Input: part model. Units: mm. Frame: model coordinates. A direction names the side the tool comes from. Round coordinates to 2 decimals unless told otherwise and drop trailing zeros. Loops run counter-clockwise (first coordinate to the right, second up) from the corner with the lowest first, then second, coordinate; pieces in that order, holes last. Notation, with made-up numbers: M 24,-25 L 73,-25 A27 cw 73,11 Z; hole C -37.5,82 d1. An arc over 180 degrees is marked long. Put each result on its own line as item: value. Start each with the question number.
1) Section C-C on x = 77.5. Output: boundary loops of the cut face in (y, z), plus the area to 3 significant figures.
2) Reachability of faces 1 (the face through (19, 30, 21.59)), 2 (the face through (0, 20, 0)), 3 (the face through (23, 32.283, -4)), 4 (the face through (95, 30, -21.59)) from +Z, -Z, +X, -X, +Y, -Y: full face, straight path, thin tool, end or side. Return the list, or none.
3) Draft query along Y for faces 5 (the face through (91.58, 34.45, 4.73)), 6 (the face through (57, -2.82, 8)), 7 (the face through (95, 27.914, 0)). Return one class per face: +Y half, -Y half, draft (parallel to the pull), parting line (faces both ways), or undercut.
4) Line query: probe 1 along Z at (x, y) = (25, 17); probe 2 along Z at (x, y) = (29, 28.5); probe 3 along Y at (x, z) = (96, -24). Output: solid intervals per line, ascending.
5) Section D-D on x = 39.5. Output: boundary loops of the cut face in (y, z).
6) Pin query (flat end, axial travel): pin 1 (19 mm diameter, centred on x = 88.9, z = 0, fed in from -Y); pin 2 (6.5 mm diameter, centred on x = 88.9, z = 0, fed in from +Y) (1 decimal). Return the tip coordinate at first contact, or that it passes through.
7) Section A-A on y = 21.5. Output: boundary loops of the cut face in (x, z), plus the area to 3 significant figures.
8) Section B-B on z = -14. Output: boundary loops of the cut face in (x, y), plus the area to 3 significant figures.
from build123d import *

# Parameters (mm, degrees)
F0_W      = 31.75
F0_H      = 63.5
F1_DEPTH  = 114.3
F2_DEPTH  = 114.3
F4_D      = 8.334375
F4_2_D    = 8.334375
F7_DEPTH  = 7.62
F8_W      = 3.556
F8_H      = 43.18
F9_DEPTH  = 38.1
F10_START = 76.2
F10_DEPTH = 38.1
F14_R     = 8.255
F14_R_2   = 4.1671875
F15_R     = 8.255
F15_R_2   = 4.1671875
F16_DEPTH = 6.35
F17_R     = 4.1671875
F18_DEPTH = 4.2672


# Not quite as in the source:
# - a length typed as a fraction of an inch, garbled in the dataset ("3 / 203.2 mm" for 3/8 in), is restored


with BuildPart() as f1:
    # F0 (on Right) → F1 (new body)
    with BuildSketch(Plane.YZ):
        with Locations((20.6751725854, 0)):
            Rectangle(F0_W, F0_H)
    extrude(amount=F1_DEPTH)

    # F4 (through all)
    with Locations(Plane.XZ.offset(26.9498274146)):
        with Locations((25.4, 0), (88.9, 0)):
            Hole(F4_D / 2)

    # F6 (on face) → F7 (join)
    with BuildSketch(Plane.XZ.offset(-4.8001725854)):
        Polygon((57.15, -31.75), (57.15, 31.75), (31.75, 31.75), (49.53, 0.9541366414), (49.53, -31.75), align=None)
        Polygon((82.55, 31.75), (57.15, 31.75), (57.15, -31.75), (64.77, -31.75), (64.77, 0.9541366414), align=None)
    extrude(amount=F7_DEPTH)

    # F8 (on face) → F9 (cut)
    with BuildSketch(Plane.YZ):
        with Locations((29.6921725854, 0)):
            Rectangle(F8_W, F8_H)
    extrude(amount=F9_DEPTH, mode=Mode.SUBTRACT)

    # F8 (on face) → F10 (cut)
    with BuildSketch(Plane.YZ.offset(F10_START)):
        with Locations((29.6921725854, 0)):
            Rectangle(F8_W, F8_H)
    extrude(amount=F10_DEPTH, mode=Mode.SUBTRACT)

    # F12: sweep along a path in F12_path
    with BuildLine(Plane(origin=(31.75, -2.8198274146, 31.75), x_dir=(0, 0, 1), z_dir=(0, -1, 0))) as f12_path:
        Line((0, 0), (-30.7958633586, -17.78))
        Line((-30.7958633586, -17.78), (-63.5, -17.78))
    # F11 (on face) → F12 (sweep, cut)
    with BuildSketch(Plane.XY.offset(31.75)):
        Polygon((35.306, 4.8001725854), (31.75, 4.8001725854), (31.75, -2.8198274146), align=None)
    sweep(path=f12_path.line, transition=Transition.RIGHT, mode=Mode.SUBTRACT)

    # F13: sweep along a path in F13_path
    with BuildLine(Plane(origin=(82.55, -2.8198274146, 31.75), x_dir=(0, 0, -1), z_dir=(0, 1, 0))) as f13_path:
        Line((0, 0), (30.7958633586, 17.78))
        Line((30.7958633586, 17.78), (63.5, 17.78))
    # F11 (on face) → F13 (sweep, cut)
    with BuildSketch(Plane.XY.offset(31.75)):
        Polygon((78.994, 4.8001725854), (82.55, -2.8198274146), (82.55, 4.8001725854), align=None)
    sweep(path=f13_path.line, transition=Transition.RIGHT, mode=Mode.SUBTRACT)

    # F14 (on face) + F15 (on face) → F16 (cut)
    with BuildSketch(Plane.XZ.offset(-4.8001725854)):
        with Locations((25.4, 0)):
            Circle(F14_R)
        with Locations((25.4, 0)):
            Circle(F14_R_2, mode=Mode.SUBTRACT)
    with BuildSketch(Plane.XZ.offset(-4.8001725854)):
        with Locations((88.9, 0)):
            Circle(F15_R)
        with Locations((88.9, 0)):
            Circle(F15_R_2, mode=Mode.SUBTRACT)
    extrude(amount=-F16_DEPTH, mode=Mode.SUBTRACT)

    # F17 (on face) → F18 (cut)
    with BuildSketch(Plane(origin=(0, 36.5501725854, 0), x_dir=(-1, 0, 0), z_dir=(0, 1, 0))):
        Polygon((-83.4644, -3.1382451232), (-83.4644, 3.1382451232), (-88.9, 6.2764902464), (-94.3356, 3.1382451232), (-94.3356, -3.1382451232), (-88.9, -6.2764902464), align=None)
        with Locations((-88.9, 0)):
            Circle(F17_R, mode=Mode.SUBTRACT)
        Polygon((-30.8356, 3.1382451232), (-30.8356, -3.1382451232), (-25.4, -6.2764902464), (-19.9644, -3.1382451232), (-19.9644, 3.1382451232), (-25.4, 6.2764902464), align=None)
        with Locations((-25.4, 0)):
            Circle(F17_R, mode=Mode.SUBTRACT)
    extrude(amount=-F18_DEPTH, mode=Mode.SUBTRACT)


with BuildPart() as f2:
    # F0 (on Right) → F2 (new body)
    with BuildSketch(Plane.YZ):
        Polygon((-26.9498274146, -19.685), (-26.9498274146, -31.75), (4.8001725854, -31.75), (4.8001725854, 31.75), (-26.9498274146, 31.75), (-26.9498274146, 19.685), (-23.3938274146, 19.685), (-7.8998274146, 8.89), (-7.8998274146, -8.89), (-23.3938274146, -19.685), align=None)
        Polygon((-26.9498274146, 19.685), (-26.9498274146, -19.685), (-23.3938274146, -19.685), (-7.8998274146, -8.89), (-7.8998274146, 8.89), (-23.3938274146, 19.685), align=None)
    extrude(amount=F2_DEPTH)

    # F4#2 (through all)
    with Locations(Plane.XZ.offset(26.9498274146)):
        with Locations((25.4, 0), (88.9, 0)):
            Hole(F4_2_D / 2)


solid = f1.part
Geometry results:
1. outline: M -2.82,23 L 4.8,29.16 L 4.8,-31.75 L 36.55,-31.75 L 36.55,31.75 L -2.82,31.75 Z; hole M 27.91,-21.59 L 31.47,-21.59 L 31.47,21.59 L 27.91,21.59 Z
1. area: 1,910 mm²
2. face 1: -X
2. face 2: +Z, -Z, -X, +Y, -Y
2. face 3: +Y
2. face 4: +X
3. face 5: draft
3. face 6: -Y half
3. face 7: undercut
4. probe 1: z = -31.75 to -4.15, 4.15 to 31.75
4. probe 2: z = -31.75 to -21.59, 21.59 to 31.75
4. probe 3: y = 4.8 to 36.55
5. outline: M -2.82,18.33 L 4.8,24.49 L 4.8,-31.75 L 36.55,-31.75 L 36.55,31.75 L -2.82,31.75 Z
6. pin 1: stops at y = 4.8
6. pin 2: passes through
7. outline: M 0,-31.75 L 114.3,-31.75 L 114.3,31.75 L 0,31.75 Z; hole C 25.4,0 d8.33; hole C 88.9,0 d8.33
7. area: 7,150 mm²
8. outline: M 0,4.8 L 52.61,4.8 L 49.53,-2.82 L 64.77,-2.82 L 61.69,4.8 L 114.3,4.8 L 114.3,27.91 L 76.2,27.91 L 76.2,31.47 L 114.3,31.47 L 114.3,36.55 L 0,36.55 L 0,31.47 L 38.1,31.47 L 38.1,27.91 L 0,27.91 Z
8. area: 3,450 mm²
